Autodesk Inventor part; units mm, degrees
ref_plane "YZ Plane" through (0, 0, 0) normal (1, 0, 0) x (0, 1, 0)
ref_plane "XZ Plane" through (0, 0, 0) normal (0, 1, 0) x (-1, 0, 0)
ref_plane "XY Plane" through (0, 0, 0) normal (0, 0, 1) x (1, 0, 0)
sketch "Sketch2" plane through (0, 0, 0) normal (0, 1, 0) x (-1, 0, 0)
  line L0 (3.5, -5.25) -> (-3.5, -5.25)
  line L1 (-3.5, -5.25) -> (-3.5, 5.25)
  line L2 (-3.5, 5.25) -> (3.5, 5.25)
  line L3 (3.5, 5.25) -> (3.5, -5.25)
  line L4 (3.5, -5.25) -> (-3.5, 5.25) construction
  line L5 (-3.5, -5.25) -> (3.5, 5.25) construction
  point P0 (0, 0)
  dimension "d11" = 10.5
  dimension "d12" = 7
sketch "Sketch3" plane through (0, 0, 0) normal (0, 0, 1) x (1, 0, 0)
  line L0 (0, 0) -> (0, 12.75)
  line L1 (0, 12.75) -> (8.0107, 17.375)
  line L2 (8.0107, 17.375) -> (-3.3643, 37.0771)
  dimension "d13" = 12.75
  dimension "d14" = 9.25
  dimension "d15" = 120
  dimension "d16" = 22.75
  dimension "d30" = 90
sweep "Sweep1" add profiles "Sketch2" path "Sketch3"
sketch "Sketch4" plane through (-3.5, 0, 5.25) normal (0, 0, 1) x (1, 0, 0)
  line L0 (7, 0) -> (0, 0)
  circle A0 centre (3.5, 3.5) radius 1.5
  point P0 (3.5, 0)
  point P1 (3.5, 0)
  dimension "d19" = 3
  dimension "d20" = 3.5
extrude "Extrusion1" cut sketch "Sketch4" against normal blind 11.5
sketch "Sketch5" plane through (-3.5, 0, 5.25) normal (0, 0, 1) x (1, 0, 0)
  line L0 (6.7296, 18.6561) -> (16.2918, 16.0939) construction
  circle A0 centre (11.5107, 17.375) radius 2
  point P0 (3.5, 0)
  dimension "d24" = 4
extrude "Extrusion2" add sketch "Sketch5" along normal blind 13.5
fillet "Fillet2" radius 3.5 8 edges at (3.5, 0, 0) (-3.5, 0, 0) (3.5, 10.7293, 0) (-0.3332, 38.8271, 0) (12.7918, 16.0939, 0) (-3.5, 14.7707, 0) (3.2296, 18.6561, 0) (-6.3954, 35.3271, 0)
sketch "Sketch6" plane through (-1.6143, 34.046, 5.25) normal (0, 0, 1) x (0.8660254, 0.5, 0)
  circle A0 centre (-13.875, -27.2607) radius 1.5
  arc A1 (-16.9061, -25.5107) -> (-10.8439, -29.0107) centre (-13.875, -27.2607) ccw
  circle A2 centre (-13.875, -27.2607) radius 3.5
  point P0 (-15.625, -30.2918)
extrude "Extrusion3" add sketch "Sketch6" along normal blind 5
properties part number "arm"
Geometry check sheet. Reference: the model listing, model coordinates, mm. A direction names the side the tool comes from. Give positions to 0.01 mm unless a question says otherwise; leave off trailing zeros. Write each loop counter-clockwise with the first axis right and the second up, starting at its lowest first coordinate (ties: lowest second). Pieces come first, ordered by that corner, then holes. Notation, with made-up numbers: (18.5, -25.5) -> (46.5, -25.5) arc R21 ccw to (46.5, 8.5) -> close; hole circle Ø7 at (12, 34.25). An arc over 180 degrees is marked (long way). Use one line per item in the form item = value.
Item 1: Depth check by flat-ended pin: pin 1 Ø4 at (y, z) = (5, 2.5) entering from +X; pin 2 Ø4 at (x, z) = (0.5, 0) entering from +Y; pin 3 Ø2 at (y, z) = (24, 2) entering from +X. Enter the tip coordinate at first touch or a pass-through.
Results list:
pin_1 = 3.5
pin_2 = 37.54
pin_3 = 8.8
Item 2: Sectioned sample at C-C on x = 4. Enter the section's corners in (y, z).
Results list:
outline = (10.51, -5.25) -> (31.32, -5.25) -> (31.32, 5.25) -> (10.51, 5.25) -> close
Item 3: Mould release check, pull along Y, two halves, no side actions. Record for faces 1 (the cylindrical face through (1.82, 18.99, 0.07)), 2 (the flat face through (-0.762, 16.351, -0.073)), 3 (the flat face through (7.54, 13.06, 0.07)), 4 (the flat face through (3, 19, -5.25)): released by +Y, released by -Y, zero draft, split by the parting line, or undercut.
Results list:
face_1 = undercut
face_2 = undercut
face_3 = released by -Y
face_4 = zero draft
Item 4: Scan lines: line 1 (Y direction, x = -0.75, z = 4); line 2 (Z direction, x = 5, y = 15.5); line 3 (X direction, y = 3.5, z = 0). Record each from-to range of solid material in increasing order.
Results list:
line_1 = 0.08 to 2.2, 4.8 to 16.36, 25.55 to 37.44
line_2 = -5.25 to 5.25
line_3 = -3.5 to -1.5, 1.5 to 3.5
Item 5: Access from +Z, -Z, +X, -X, +Y, -Y to the whole of each face (thin tool, end or side, straight path). Record for faces 5 (the cylindrical face through (0, 7, 8)), 6 (the flat face through (8, 17, 18.75)), 7 (the cylindrical face through (7.75, 15.392, 11.906)), 8 (the flat face through (-3.5, 8, 0)), 9 (the flat face through (-1.63, 27.07, -0.07)).
Results list:
face_5 = +Z, +Y
face_6 = +Z, +X, -X, +Y, -Y
face_7 = +Z
face_8 = +Z, -Z, -X, -Y
face_9 = +Z, -Z, -X
Item 6: Sectioned sample at D-D on y = 20. Enter the section's corners in (x, z), plus the area to 3 significant figures.
Results list:
outline = (1.95, -5.25) -> (10.54, -5.25) -> (10.54, 5.25) -> (1.95, 5.25) -> close
area = 90.2 mm2
Item 7: Sectioned sample at B-B on x = -0.75. Enter the section's corners in (y, z), plus the area to 3 significant figures.
Results list:
outline = (0.08, -5.25) -> (2.2, -5.25) -> (2.2, 10.25) -> (0.08, 10.25) -> close; (4.8, -5.25) -> (16.36, -5.25) -> (16.36, 5.25) -> (6.92, 5.25) -> (6.92, 10.25) -> (4.8, 10.25) -> close; (25.55, -5.25) -> (37.44, -5.25) -> (37.44, 5.25) -> (25.55, 5.25) -> close
area = 290 mm2
